For this review, take the finished solid that the model builds, in its own axes (mm). Face numbers are marked on the shaded views. A direction names the side the tool comes from. Coordinates: 2 decimals unless noted, no trailing zeros. Write each loop counter-clockwise with the first axis right and the second up, starting at its lowest first coordinate (ties: lowest second). Pieces come first, ordered by that corner, then holes.
1) To check wall thickness, follow line 1 along Y through (x, z) = (-24, 10.5); line 2 along X through (y, z) = (-5.25, 8.25); line 3 along Z through (x, y) = (20, 1.5). State the ranges of each line that lie inside material, in increasing order.
2) Insertion check: P1, Ø9, axis at x = 24, y = 0, coming from the +Z side; P2, Ø8, axis at x = 0, z = 9, coming from the +Y side. Each pin has a flat end and moves straight along its axis. Give the tip position at first contact, or say it passes through.
3) We need section A-A on z = 9. Write out the cut boundary in (x, y).
4) For the marked faces 4, 5 and 6, list the 3-axis set-ups (+Z, -Z, +X, -X, +Y, -Y) from which the entire face can be reached by the end or side of a thin tool; tool diameter is ignored.
5) We need section C-C on y = 0. Write out the cut boundary in (x, z).
6) We need section D-D on x = 24. Write out the cut boundary in (y, z), then the cut area to 3 significant figures.
7) We need section B-B on x = 0. Write out the cut boundary in (y, z).
8) Mouldability with a two-part tool opening along Y and no side actions: class the marked faces 1, 2 and 3 as pulls with the +Y half, pulls with the -Y half, needs draft (parallel to the pull), parting line crosses it, or undercut.
from build123d import *

# Parameters (mm, degrees)
SKETCH1_W           = 75
SKETCH1_H           = 25
BOSS_EXTRUDE1_DEPTH = 18
SKETCH2_R           = 7.5
CUT_EXTRUDE1_DEPTH  = 10
SKETCH3_R           = 2.5
CUT_EXTRUDE2_DEPTH  = 49.53091798
SKETCH4_R           = 5
CUT_EXTRUDE3_DEPTH  = 6


with BuildPart() as part:
    # Sketch1 → Boss-Extrude1 (new body)
    with BuildSketch(Plane.XY):
        Rectangle(SKETCH1_W, SKETCH1_H)
    extrude(amount=BOSS_EXTRUDE1_DEPTH)

    # Sketch2 → Cut-Extrude1 (cut)
    with BuildSketch(Plane.XY.offset(18)):
        with Locations((-24, 0)):
            Circle(SKETCH2_R)
        with Locations((24, 0)):
            Circle(SKETCH2_R)
    extrude(amount=-CUT_EXTRUDE1_DEPTH, mode=Mode.SUBTRACT)

    # Sketch3 → Cut-Extrude2 (cut, through all)
    with BuildSketch(Plane.XZ.offset(12.5)):
        with Locations(Location((0, 9, 0), (0, 0, 270))):
            Circle(SKETCH3_R)
    extrude(amount=-CUT_EXTRUDE2_DEPTH, mode=Mode.SUBTRACT)

    # Sketch4 → Cut-Extrude3 (cut)
    with BuildSketch(Plane(origin=(0, 12.5, 0), x_dir=(1, 0, 0), z_dir=(0, 1, 0))):
        with Locations(Location((0, -9, 0), (0, 0, 270))):
            Circle(SKETCH4_R)
    extrude(amount=-CUT_EXTRUDE3_DEPTH, mode=Mode.SUBTRACT)


solid = part.part
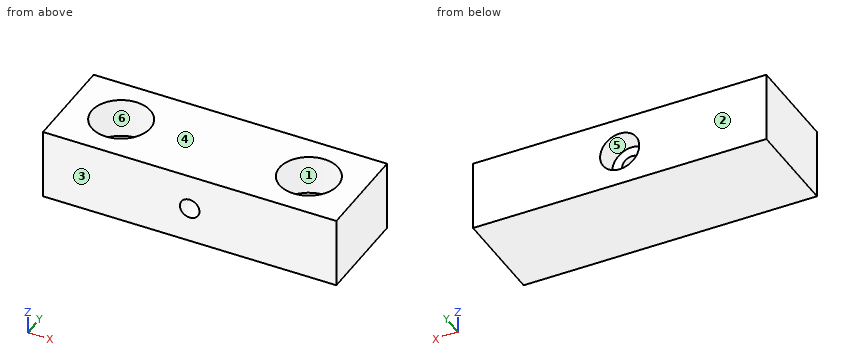
Result:
1. line 1: y = -12.5 to -7.5, 7.5 to 12.5
1. line 2: x = -37.5 to -29.36, -18.64 to -2.38, 2.38 to 18.64, 29.36 to 37.5
1. line 3: z = 0 to 8
2. P1: stops at z = 8
2. P2: stops at y = 6.5
3. outline: (-37.5, -12.5) - (-2.5, -12.5) - (-2.5, 6.5) - (-5, 6.5) - (-5, 12.5) - (-37.5, 12.5) - close; (2.5, -12.5) - (37.5, -12.5) - (37.5, 12.5) - (5, 12.5) - (5, 6.5) - (2.5, 6.5) - close; hole circle Ø15 at (-24, 0); hole circle Ø15 at (24, 0)
4. face 4: +Z, +X, -X, +Y, -Y
4. face 5: +Y
4. face 6: +Z
5. outline: (-37.5, 0) - (37.5, 0) - (37.5, 18) - (31.5, 18) - (31.5, 8) - (16.5, 8) - (16.5, 18) - (-16.5, 18) - (-16.5, 8) - (-31.5, 8) - (-31.5, 18) - (-37.5, 18) - close; hole circle Ø5 at (0, 9)
6. outline: (-12.5, 0) - (12.5, 0) - (12.5, 18) - (7.5, 18) - (7.5, 8) - (-7.5, 8) - (-7.5, 18) - (-12.5, 18) - close
6. area: 300 mm2
7. outline: (-12.5, 0) - (12.5, 0) - (12.5, 4) - (6.5, 4) - (6.5, 6.5) - (-12.5, 6.5) - close; (-12.5, 11.5) - (6.5, 11.5) - (6.5, 14) - (12.5, 14) - (12.5, 18) - (-12.5, 18) - close
8. face 1: undercut
8. face 2: pulls with the +Y half
8. face 3: pulls with the -Y half
